```python
from build123d import *

# Parameters (mm, degrees)
T_LE_DE_BASE_PLI_E1_DEPTH                      = 72.5
CONG_1_R                                       = 2
FRAISAGE_POUR_VIS_T_TE_FRAIS_E_M31_D           = 3.4
FRAISAGE_POUR_VIS_T_TE_FRAIS_E_M31_CSINK_D     = 6.3
FRAISAGE_POUR_VIS_T_TE_FRAIS_E_M31_CSINK_ANGLE = 90
T_LE_PLI_E_SUR_AR_TE1_DEPTH                    = 52
CONG_2_R                                       = 1


# Sheet-metal steps are written as plain solids
with BuildPart() as part:
    # Esquisse1 → Tôle de base pliée1 (new body)
    with BuildSketch(Plane.XY):
        with BuildLine():
            Line((0, 0), (74.252230641, 0))
            ThreePointArc((74.252230641, 0), (74.952645404, 0.126655622), (75.564348699, 0.49058084))
            Line((75.564348699, 0.49058084), (95.377158666, 17.713593783))
            Line((95.377158666, 17.713593783), (96.36124721, 16.581529412))
            Line((96.36124721, 16.581529412), (76.548437242, -0.641483531))
            ThreePointArc((76.548437242, -0.641483531), (75.477956475, -1.278352662), (74.252230641, -1.5))
            Line((74.252230641, -1.5), (0, -1.5))
            Line((0, -1.5), (0, 0))
        make_face()
    extrude(amount=T_LE_DE_BASE_PLI_E1_DEPTH)

    # Congé1
    cong_1_edges = [part.edges().sort_by_distance(p)[0] for p in [
        (0, -0.75, 72.5),
        (95.869202938, 17.147561598, 72.5),
        (0, -0.75, 0),
        (95.869202938, 17.147561598, 0),
    ]]
    fillet(cong_1_edges, radius=CONG_1_R)

    # Fraisage pour vis à tête fraisée M31 (through all)
    with Locations(Plane(origin=(33.265097257, -38.267116948, 0), x_dir=(0, 0, -1), z_dir=(0.6560590289905085, -0.7547095802227711, 0))):
        with Locations((-56.25, 77.603218517), (-16.25, 77.603218517)):
            CounterSinkHole(FRAISAGE_POUR_VIS_T_TE_FRAIS_E_M31_D / 2, FRAISAGE_POUR_VIS_T_TE_FRAIS_E_M31_CSINK_D / 2, counter_sink_angle=FRAISAGE_POUR_VIS_T_TE_FRAIS_E_M31_CSINK_ANGLE)

    # Tôle pliée sur arête1 section (across the edge) → Tôle pliée sur arête1 (add)
    with BuildSketch(Plane(origin=(65.252230641, 0, -2), x_dir=(0, 0, 1), z_dir=(-1, 0, 0))):
        with BuildLine():
            Line((-1.5, 2), (-1.5, 9))
            Line((-1.5, 9), (0, 9))
            Line((0, 9), (0, 2))
            ThreePointArc((0, 2), (0.585786438, 0.585786438), (2, 0))
            Line((2, 0), (2, -1.5))
            ThreePointArc((2, -1.5), (-0.474873734, -0.474873734), (-1.5, 2))
        make_face()
    extrude(amount=T_LE_PLI_E_SUR_AR_TE1_DEPTH)

    # Congé2
    cong_2_edges = [part.edges().sort_by_distance(p)[0] for p in [
        (65.252230641, 9, -2.75),
        (13.252230641, 9, -2.75),
    ]]
    fillet(cong_2_edges, radius=CONG_2_R)


solid = part.part
```
Can you work these out from the model? Positions are in its coordinate system, mm. A direction names the side the tool comes from. Give positions to 0.01 mm unless a question says otherwise; leave off trailing zeros. Order: outer loops, then holes, each group sorted by start corner. A loop starts at its lowest first (then second) coordinate and runs counter-clockwise, first axis right, second up. Notation, with made-up numbers: M 25,20 L 49,20 A18 ccw 49,42 Z; hole C -24,89 d10. An arc over 180 degrees is marked long. Write item = value, one per line. Start each with the question number.
Q1. Suppose I cut it at C-C (x = 22.5). Write out the boundary of the cut face in (y, z), plus the area to 3 significant figures.
Q2. Will these pins go through, and if not, where does the flat tip stop? pin 1 Ø10 at (y, z) = (12, 36) entering from +X; pin 2 Ø5.5 at (x, y) = (83, 6.5) entering from -Z; pin 3 Ø6 at (y, z) = (8, 64.5) entering from +X.
Q3. Suppose I cut it at D-D (x = 7). Write out the boundary of the cut face in (y, z), plus the area to 3 significant figures.
Q4. I need wall thicknesses on probe 1 along Y at (x, z) = (7.5, 10); probe 2 along Z at (x, y) = (53, 7); probe 3 along X at (y, z) = (1, 19). Which ranges of each line are inside material? Lowest first, please. Write a range as [from, to].
Q5. For faces 1 (the flat face through (40, 6, -2)), 2 (the flat face through (13.252, 3, -3)), 3 (the flat face through (37, 0, 36)), 4 (the flat face through (65.252, 3, -3)), which set-ups out of +Z, -Z, +X, -X, +Y, -Y let a thin tool reach every point of the face, with its end or its side?
Q6. Suppose I cut it at B-B (z = 24.5). Write out the boundary of the cut face in (x, y).
Q7. Suppose I cut it at A-A (y = 3). Write out the boundary of the cut face in (x, z).
Check result:
q1.outline = M -1.5,0 A3.5 ccw 2,-3.5 L 9,-3.5 L 9,-2 L 2,-2 A2 cw 0,0 L 0,72.5 L -1.5,72.5 Z
q1.area = 126 mm2
q2.pin_1 = 96.36
q2.pin_2 = 0
q2.pin_3 = 89.94
q3.outline = M -1.5,0 L 0,0 L 0,72.5 L -1.5,72.5 Z
q3.area = 109 mm2
q4.probe_1 = [-1.5, 0]
q4.probe_2 = [-3.5, -2]
q4.probe_3 = [76.15, 78.44]
q5.face_1 = +Z, +X, -X, +Y
q5.face_2 = -Z, -X, +Y, -Y
q5.face_3 = +Z, -X, +Y
q5.face_4 = -Z, +X, +Y, -Y
q6.outline = M 0,-1.5 L 74.25,-1.5 A3.5 ccw 76.55,-0.64 L 96.36,16.58 L 95.38,17.71 L 75.56,0.49 A2 cw 74.25,0 L 0,0 Z
q7.outline = M 13.25,-3.5 L 65.25,-3.5 L 65.25,-2 L 13.25,-2 Z; M 78.45,0 L 80.74,0 L 80.74,72.5 L 78.45,72.5 Z
